Work out the finished part from the listing and answer in its coordinate system (mm). A direction names the side the tool comes from. Round coordinates to 2 decimals unless told otherwise and drop trailing zeros. Write each loop counter-clockwise with the first axis right and the second up, starting at its lowest first coordinate (ties: lowest second). Pieces come first, ordered by that corner, then holes. Notation, with made-up numbers: (73, 53.5) - (78, 53.5) arc R19 cw to (78, 60.5) - close; hole circle Ø7 at (64.5, 4). An arc over 180 degrees is marked (long way). Answer as a JSON object with one key per item and string values.
Solid Edge part; units mm, degrees
sketch "Sketch1" plane through (0, 0, 0) normal (0, 0, 1) x (1, 0, 0)
  line L0 (-60, 29) -> (60, 29)
  line L1 (60, 29) -> (60, -29)
  line L2 (60, -29) -> (-60, -29)
  line L3 (-60, -29) -> (-60, 29)
  dimension "D1" = 60
  dimension "D2" = 60
extrude "Protrusion1" add sketch "Sketch1" along normal blind 30
fillet "Redondo_1" radius 2 4 edges at (60, 29, 15) (60, -29, 15) (-60, 29, 15) (-60, -29, 15)
sketch "Sketch2" plane through (0, 0, 0) normal (0, 0, -1) x (-1, 0, 0)
  line L0 (-56, 27.0038) -> (56, 27.0038)
  arc A0 (56, 27.0038) -> (58, 25.0038) centre (56, 25.0038) cw
  line L1 (58, 25.0038) -> (58, -24.9962)
  arc A1 (56, -26.9962) -> (58, -24.9962) centre (56, -24.9962) ccw
  line L2 (56, -26.9962) -> (-56, -26.9962)
  arc A2 (-56, -26.9962) -> (-58, -24.9962) centre (-56, -24.9962) cw
  line L3 (-58, -24.9962) -> (-58, 25.0038)
  arc A3 (-56, 27.0038) -> (-58, 25.0038) centre (-56, 25.0038) ccw
extrude "Cutout1" cut sketch "Sketch2" against normal blind 28
sketch "Sketch3" plane through (60, 0, 15) normal (1, 0, 0) x (0, 1, 0)
  circle A0 centre (19.8269, -3.4527) radius 1.5502
  circle A1 centre (-20.1684, -3.3569) radius 1.5502
  line L0 (14.8624, 1.8687) -> (14.8624, -8.466)
  arc A2 (14.8624, -8.466) -> (8.3284, -15) centre (8.3284, -8.466) cw
  line L1 (-8.8017, -15) -> (8.3284, -15)
  arc A3 (-8.8017, -15) -> (-15.1376, -8.6641) centre (-8.8017, -8.6641) cw
  line L2 (-15.1376, -8.6641) -> (-15.1376, 1.5062)
  arc A4 (-15.1376, 1.5062) -> (-8.8438, 7.8) centre (-8.8438, 1.5062) cw
  line L3 (8.9311, 7.8) -> (-8.8438, 7.8)
  arc A5 (8.9311, 7.8) -> (14.8624, 1.8687) centre (8.9311, 1.8687) cw
extrude "Recorte_Extrudado_3" cut sketch "Sketch3" against normal blind 5
sketch "Sketch4" plane through (-60, 0, 15) normal (-1, 0, 0) x (0, -1, 0)
  line L0 (-7.2229, -2.44) -> (-22.9734, -2.44)
  line L1 (-22.8392, -15) -> (-22.9734, -2.44)
  line L2 (-7.2229, -15) -> (-22.8392, -15)
  line L3 (-7.2229, -2.44) -> (-7.2229, -15)
  line L4 (23.2376, -2.377) -> (7.6078, -2.377)
  line L5 (7.6078, -2.377) -> (7.5447, -15)
  line L6 (7.5447, -15) -> (23.2376, -15)
  line L7 (23.2376, -2.377) -> (23.2376, -15)
extrude "Recorte_Extrudado_4" cut sketch "Sketch4" against normal blind 4
Item 1: A cutting plane is placed at C-C (y = 0.5). Write down the section's boundary in (x, z), and give its area (3 significant figures).
Results found:
{"outline": "(-60, 0) - (-58, 0) - (-58, 28) - (58, 28) - (58, 22.8) - (60, 22.8) - (60, 30) - (-60, 30) - close", "area": "306 mm²"}
Item 2: For faces 4 (the cylindrical face through (59.01, -13.24, 21.01)), 5 (the flat face through (-1, 0, 28)), 6 (the cylindrical face through (59.014, -13.331, 1.905)), 7 (the flat face through (1, -29, 15)), determine the directions among +Z, -Z, +X, -X, +Y, -Y from which every point of the face is accessible in a straight line to the end or side of a thin tool.
Results found:
{"face 4": "+X", "face 5": "-Z", "face 6": "+X, -X", "face 7": "+Z, -Z, +X, -X, -Y"}
Item 3: Each of these flat-tipped pins is pushed along its axis until it touches: P1, Ø3, axis at y = -20.17, z = 11.64, coming from the +X side; P2, Ø1.6, axis at x = -59, y = 14, coming from the -Z side; P3, Ø1, axis at x = 59.5, y = 3.5, coming from the -Z side. Where does it stop, or does it pass through?
Results found:
{"P1": "x = -58", "P2": "z = 12.56", "P3": "z = 22.8"}
Item 4: A cutting plane is placed at B-B (x = 52.5). Write down the section's boundary in (y, z), and give its area (3 significant figures).
Results found:
{"outline": "(-29, 0) - (-27, 0) - (-27, 28) - (27, 28) - (27, 0) - (29, 0) - (29, 30) - (-29, 30) - close", "area": "228 mm²"}
Item 5: A cutting plane is placed at D-D (z = 4). Write down the section's boundary in (x, y).
Results found:
{"outline": "(-60, -27) arc R2 ccw to (-58, -29) - (58, -29) arc R2 ccw to (60, -27) - (60, -14.69) - (58, -14.69) - (58, -25) arc R2 cw to (56, -27) - (-56, -27) arc R2 cw to (-58, -25) - (-58, -23.24) - (-60, -23.24) - close; (-60, -7.56) - (-58, -7.56) - (-58, 7.22) - (-60, 7.22) - close; (-60, 22.88) - (-58, 22.88) - (-58, 25) arc R2 cw to (-56, 27) - (56, 27) arc R2 cw to (58, 25) - (58, 14.35) - (60, 14.35) - (60, 27) arc R2 ccw to (58, 29) - (-58, 29) arc R2 ccw to (-60, 27) - close"}
Item 6: A cutting plane is placed at A-A (z = 25.5). Write down the section's boundary in (x, y), and give its area (3 significant figures).
Results found:
{"outline": "(-60, -27) arc R2 ccw to (-58, -29) - (58, -29) arc R2 ccw to (60, -27) - (60, 27) arc R2 ccw to (58, 29) - (-58, 29) arc R2 ccw to (-60, 27) - close; hole (-58, -25) arc R2 ccw to (-56, -27) - (56, -27) arc R2 ccw to (58, -25) - (58, 25) arc R2 ccw to (56, 27) - (-56, 27) arc R2 ccw to (-58, 25) - close", "area": "696 mm²"}
Item 7: Consider line 1 along X through (y, z) = (-19, 20); line 2 along Y through (x, z) = (52, 21.5); line 3 along Z through (x, y) = (25.5, 3.5). Determine where each line is inside the solid, lowest interval first.
Results found:
{"line 1": "-60 to -58, 58 to 60", "line 2": "-29 to -27, 27 to 29", "line 3": "28 to 30"}
Item 8: Determine the mould class of faces 1 (the flat face through (14, 28, 0)), 2 (the cylindrical face through (59.01, 13.17, 21.02)), 3 (the flat face through (-58, 0, 17)) for opening direction Z: pulls with the +Z half, pulls with the -Z half, needs draft (parallel to the pull), parting line crosses it, or undercut.
Results found:
{"face 1": "pulls with the -Z half", "face 2": "undercut", "face 3": "needs draft"}
